Design review of the part built by this model. Coordinates are the model's own, in mm. Round coordinates to 2 decimals unless told otherwise and drop trailing zeros. Write each loop counter-clockwise with the first axis right and the second up, starting at its lowest first coordinate (ties: lowest second). Pieces come first, ordered by that corner, then holes. Notation, with made-up numbers: M 48.5,-15.5 L 80.5,-15.5 A5 cw 80.5,-11.5 Z; hole C 86.25,1.5 d2. An arc over 180 degrees is marked long. One line per question, with ' | ' between items. Start each with the question number.
Item 1: Add section D-D, the plane y = 13.75. State the section outline as (x, z) points (3 decimals).
Item 2: Draft analysis for pull direction X (two halves, no side actions). For faces 1 (the face through (15.88, 10.4, -0.14)), 2 (the face through (25.4, 10, 0)), 3 (the face through (-0.28, 12.57, -0.18)), 4 (the face through (0, 20.51, 0)), state which applies: released by +X, released by -X, zero draft, split by the parting line, or undercut.
Item 3: For L1, parallel to Z at x = 19.05, y = 5.25 (3 decimals); L2, parallel to X at y = 6.75, z = 2.75; L3, parallel to X at y = 17, z = -2.25, list the stretches that pass through material, from the lowest coordinate up.
Item 4: Add section C-C, the plane x = -19.05. State the section outline as (y, z) points (1 decimal), and give its area (3 significant figures).
Item 5: Add section A-A, the plane z = 0. State the section outline as (x, y) points (1 decimal), and give its area (3 significant figures).
Item 6: Insertion check: pin 1 Ø5 at (x, z) = (10.5, 3) entering from -Y. The pin has a flat end and moves straight along its axis. Give the tip position at first contact, or say it passes through.
Item 7: Add section B-B, the plane y = 8. State the section outline as (x, z) points (3 decimals).
```python
from build123d import *

# Parameters (mm, degrees)
SKETCH1_W        = 50.8
SKETCH1_H        = 25.4
BLOCK_DEPTH      = 20.5105
SKETCH3_R        = 12.7
SHAFT_HOLE_DEPTH = 42.364243136
CLAMPING_HOLES_D = 6.35


with BuildPart() as part:
    # Sketch1 → Block (new body)
    with BuildSketch(Plane(origin=(0, 0, 0), x_dir=(1, 0, 0), z_dir=(0, 1, 0))):
        Rectangle(SKETCH1_W, SKETCH1_H)
    extrude(amount=BLOCK_DEPTH)

    # Sketch3 → Shaft Hole (cut, through all)
    with BuildSketch(Plane(origin=(0, 0, -12.7), x_dir=(-1, 0, 0), z_dir=(0, 0, -1))):
        with Locations((0, -0.127)):
            Circle(SKETCH3_R)
    extrude(amount=-SHAFT_HOLE_DEPTH, mode=Mode.SUBTRACT)

    # Clamping Holes (through all)
    with Locations(Plane(origin=(0, 0, 0), x_dir=(-1, 0, 0), z_dir=(0, -1, 0))):
        with Locations((-19.05, 0), (19.05, 0)):
            Hole(CLAMPING_HOLES_D / 2)


solid = part.part
```
Computed values:
1) outline: M -25.4,-12.7 L 25.4,-12.7 L 25.4,12.7 L -25.4,12.7 Z; hole C -19.05,0 d6.35; hole C 19.05,0 d6.35
2) face 1: undercut | face 2: released by +X | face 3: undercut | face 4: zero draft
3) L1: z = -12.7 to -3.175, 3.175 to 12.7 | L2: x = -25.4 to -20.64, -17.46 to -10.68, 10.68 to 17.46, 20.64 to 25.4 | L3: x = -25.4 to -21.29, -16.81 to 16.81, 21.29 to 25.4
4) outline: M 0,-12.7 L 20.5,-12.7 L 20.5,-3.2 L 0,-3.2 Z; M 0,3.2 L 20.5,3.2 L 20.5,12.7 L 0,12.7 Z | area: 391 mm^2
5) outline: M -25.4,0 L -22.2,0 L -22.2,20.5 L -25.4,20.5 Z; M -15.9,0 L -12.7,0 A12.7 cw 12.7,0 L 15.9,0 L 15.9,20.5 L -15.9,20.5 Z; M 22.2,0 L 25.4,0 L 25.4,20.5 L 22.2,20.5 Z | area: 531 mm^2
6) pin 1: stops at y = 0
7) outline: M -25.4,-12.7 L -9.759,-12.7 L -9.759,12.7 L -25.4,12.7 Z; M 9.759,-12.7 L 25.4,-12.7 L 25.4,12.7 L 9.759,12.7 Z; hole C -19.05,0 d6.35; hole C 19.05,0 d6.35
